Could you check a few things on this model? Use its own coordinates, in mm. A direction names the side the tool comes from. Round coordinates to 2 decimals unless told otherwise and drop trailing zeros. Loops run counter-clockwise (first coordinate to the right, second up) from the corner with the lowest first, then second, coordinate; pieces in that order, holes last.
from build123d import *

# Parameters (mm, degrees)
SKETCH1_W           = 180
SKETCH1_H           = 180
SKETCH1_R           = 10
BOSS_EXTRUDE1_DEPTH = 40
SKETCH2_R           = 23
CUT_EXTRUDE1_DEPTH  = 5
SKETCH3_R           = 25
CUT_EXTRUDE2_DEPTH  = 18
SKETCH4_R           = 12.5
CUT_EXTRUDE3_DEPTH  = 18


with BuildPart() as part:
    # Sketch1 → Boss-Extrude1 (new body)
    with BuildSketch(Plane(origin=(0, 0, 0), x_dir=(1, 0, 0), z_dir=(0, 1, 0))):
        Rectangle(SKETCH1_W, SKETCH1_H)
        with Locations(Location((-70, 70, 0), (0, 0, 270))):
            Circle(SKETCH1_R, mode=Mode.SUBTRACT)
        with Locations(Location((70, 70, 0), (0, 0, 270))):
            Circle(SKETCH1_R, mode=Mode.SUBTRACT)
        with Locations(Location((-70, -70, 0), (0, 0, 270))):
            Circle(SKETCH1_R, mode=Mode.SUBTRACT)
        with Locations(Location((70, -70, 0), (0, 0, 270))):
            Circle(SKETCH1_R, mode=Mode.SUBTRACT)
    extrude(amount=BOSS_EXTRUDE1_DEPTH)

    # Sketch2 → Cut-Extrude1 (cut)
    with BuildSketch(Plane(origin=(0, 40, 0), x_dir=(1, 0, 0), z_dir=(0, 1, 0))):
        with Locations(Location((0, 0, 0), (0, 0, 270))):
            Circle(SKETCH2_R)
    extrude(amount=-CUT_EXTRUDE1_DEPTH, mode=Mode.SUBTRACT)

    # Sketch3 → Cut-Extrude2 (cut)
    with BuildSketch(Plane.XZ):
        with Locations(Location((0, 0, 0), (0, 0, 270))):
            Circle(SKETCH3_R)
    extrude(amount=-CUT_EXTRUDE2_DEPTH, mode=Mode.SUBTRACT)

    # Sketch4 → Cut-Extrude3 (cut)
    with BuildSketch(Plane.XZ.offset(-18)):
        with Locations(Location((0, 0, 0), (0, 0, 270))):
            Circle(SKETCH4_R)
    extrude(amount=-CUT_EXTRUDE3_DEPTH, mode=Mode.SUBTRACT)


solid = part.part
Item 1: If we section it at C-C, the plane x = -70: Please give me the cut outline in (y, z), then the cut area to 3 significant figures.
Results list:
outline: (0, -90) - (40, -90) - (40, -80) - (0, -80) - close; (0, -60) - (40, -60) - (40, 60) - (0, 60) - close; (0, 80) - (40, 80) - (40, 90) - (0, 90) - close
area: 5,600 mm2
Item 2: We'd pull the mould along Z, two halves only. Please class faces 1 (the cylindrical face through (7.509, 8.874, -23.846)), 2 (the flat face through (-1, 20, 90)), 3 (the flat face through (90, 20, 1)): released by +Z, released by -Z, zero draft, split by the parting line, or undercut.
Results list:
face 1: undercut
face 2: released by +Z
face 3: zero draft
Item 3: Will this pin go through, and if not, where does the flat tip stop? pin 1 (16 mm diameter, centred on x = -70, z = 70, fed in from -Y).
Results list:
pin 1: passes through
Item 4: For faces 4 (the cylindrical face through (19.394, 37.535, 12.365)), 5 (the cylindrical face through (70, 20, 60)), 6 (the flat face through (5.9, 18, 11.5)), which set-ups out of +Z, -Z, +X, -X, +Y, -Y let a thin tool reach every point of the face, with its end or its side?
Results list:
face 4: +Y
face 5: +Y, -Y
face 6: -Y
Item 5: If we section it at D-D, the plane y = 25: Please give me the cut outline in (x, z).
Results list:
outline: (-90, -90) - (90, -90) - (90, 90) - (-90, 90) - close; hole circle Ø20 at (-70, -70); hole circle Ø20 at (-70, 70); hole circle Ø25 at (0, 0); hole circle Ø20 at (70, -70); hole circle Ø20 at (70, 70)
Item 6: If we section it at A-A, the plane z = 70: Please give me the cut outline in (x, y), then the cut area to 3 significant figures.
Results list:
outline: (-90, 0) - (-80, 0) - (-80, 40) - (-90, 40) - close; (-60, 0) - (60, 0) - (60, 40) - (-60, 40) - close; (80, 0) - (90, 0) - (90, 40) - (80, 40) - close
area: 5,600 mm2
Item 7: If we section it at B-B, the plane x = 0: Please give me the cut outline in (y, z).
Results list:
outline: (0, -90) - (40, -90) - (40, -23) - (35, -23) - (35, -12.5) - (18, -12.5) - (18, -25) - (0, -25) - close; (0, 25) - (18, 25) - (18, 12.5) - (35, 12.5) - (35, 23) - (40, 23) - (40, 90) - (0, 90) - close
Item 8: If I drill on line 1 along X through (y, z) = (13.5, 70); line 2 along X through (y, z) = (23, -61); line 3 along X through (y, z) = (37, 0), over which ranges is the centre line in solid material (lowest first)?
Results list:
line 1: x = -90 to -80, -60 to 60, 80 to 90
line 2: x = -90 to -74.36, -65.64 to 65.64, 74.36 to 90
line 3: x = -90 to -23, 23 to 90
